```python
from build123d import *

# Parameters (mm, degrees)
BOSS_EXTRUDE3_DEPTH = 101.6


with BuildPart() as part:
    # Sketch3 → Boss-Extrude3 (new body)
    with BuildSketch(Plane.XY):
        with BuildLine():
            Line((63.5, 0), (60.96, 0))
            ThreePointArc((60.96, 0), (53.713522989, -28.826707202), (33.69690787, -50.8))
            ThreePointArc((33.69690787, -50.8), (0, -60.96), (-33.69690787, -50.8))
            ThreePointArc((-33.69690787, -50.8), (-53.713522989, -28.826707202), (-60.96, 0))
            Line((-60.96, 0), (-63.5, 0))
            ThreePointArc((-63.5, 0), (0, -63.5), (63.5, 0))
        make_face()
        with BuildLine():
            ThreePointArc((-33.69690787, -50.8), (0, -60.96), (33.69690787, -50.8))
            Line((33.69690787, -50.8), (-33.69690787, -50.8))
        make_face()
    extrude(amount=BOSS_EXTRUDE3_DEPTH)


solid = part.part
```
The model under review builds one solid part; all positions refer to its coordinate system, in mm. A direction names the side the tool comes from. Round coordinates to 2 decimals unless told otherwise and drop trailing zeros. Loops run counter-clockwise (first coordinate to the right, second up) from the corner with the lowest first, then second, coordinate; pieces in that order, holes last. Notation, with made-up numbers: M 35,11.5 L 61,11.5 A23 cw 61,22.5 Z; hole C -38,-26 d1. An arc over 180 degrees is marked long. Write item = value, one per line.
Item 1: Take a section at A-A on y = -7.5. Write out the cut boundary in (x, z), then the cut area to 3 significant figures.
Return value:
outline = M -63.06,0 L -60.5,0 L -60.5,101.6 L -63.06,101.6 Z; M 60.5,0 L 63.06,0 L 63.06,101.6 L 60.5,101.6 Z
area = 520 mm2
Item 2: Take a section at D-D on y = -42. Write out the cut boundary in (x, z).
Return value:
outline = M -47.63,0 L -44.18,0 L -44.18,101.6 L -47.63,101.6 Z; M 44.18,0 L 47.63,0 L 47.63,101.6 L 44.18,101.6 Z
Item 3: Insertion check: P1, Ø2, axis at x = 6, z = 57, coming from the +Y side; P2, Ø1.5, axis at y = -54, z = 15.5, coming from the +X side; P3, Ø8, axis at y = -17, z = 65.5, coming from the -X side. Each pin has a flat end and moves straight along its axis. Give the tip position at first contact, or say it passes through.
Return value:
P1 = -50.8
P2 = 34.59
P3 = -62.16
Item 4: Take a section at B-B on z = 78. Write out the cut boundary in (x, y), then the cut area to 3 significant figures.
Return value:
outline = M -63.5,0 A63.5 ccw 63.5,0 L 60.96,0 A60.96 cw 33.7,-50.8 L -33.7,-50.8 A60.96 cw -60.96,0 Z
area = 961 mm2
Item 5: Take a section at C-C on x = 0. Write out the cut boundary in (y, z).
Return value:
outline = M -63.5,0 L -50.8,0 L -50.8,101.6 L -63.5,101.6 Z
Item 6: For line 1 (X direction, y = -48, z = 57.5); line 2 (X direction, y = -35, z = 88); line 3 (Y direction, x = 34.5, z = 7), list the stretches that pass through material, from the lowest coordinate up. Write a range as [from, to].
Return value:
line_1 = [-41.57, -37.58], [37.58, 41.57]
line_2 = [-52.98, -49.91], [49.91, 52.98]
line_3 = [-53.31, -50.26]
Item 7: Machinability: for faces 4 (the flat face through (0, -53, 101.6)), 5 (the flat face through (0, -50.8, 50)), which of the approach directions +Z, -Z, +X, -X, +Y, -Y give a long, thin tool a straight path to every point of the face, cutting with its end or side? Answer none if there is none.
Return value:
face_4 = +Z, +X, -X, +Y, -Y
face_5 = +Z, -Z, +Y
Item 8: The part is to be moulded in two halves that separate along X. For faces 1 (the flat face through (0, -53, 0)), 2 (the cylindrical face through (-1.396, -63.485, 50.089)), 3 (the cylindrical face through (-53.51, -29.2, 50.09)), say which applies: released by +X, released by -X, zero draft, split by the parting line, or undercut.
Return value:
face_1 = zero draft
face_2 = split by the parting line
face_3 = undercut
